For this review, take the finished solid that the model builds, in its own axes (mm). A direction names the side the tool comes from. Round coordinates to 2 decimals unless told otherwise and drop trailing zeros. Loops run counter-clockwise (first coordinate to the right, second up) from the corner with the lowest first, then second, coordinate; pieces in that order, holes last.
1) Take a section at D-D (x = 68.5). State the section outline as (y, z) points.
2) Take a section at B-B (z = 8.25). State the section outline as (x, y) points.
3) Tool access review of faces 1 (the flat face through (20.434, 20.28, 4.93)), 2 (the flat face through (64, 100, 5)), 3 (the flat face through (59, 80, 5)): name each direction out of +Z, -Z, +X, -X, +Y, -Y from which nothing blocks a thin tool from reaching the whole face with its end or side.
4) Take a section at C-C (y = 34). State the section outline as (x, z) points.
5) Mouldability with a two-part tool opening along Y and no side actions: class faces 4 (the flat face through (49, 51, 10)), 5 (the flat face through (8, 0, 5)), 6 (the flat face through (33.72, 69.86, 4.93)) as pulls with the +Y half, pulls with the -Y half, needs draft (parallel to the pull), parting line crosses it, or undercut.
6) Take a section at A-A (x = 55.5). State the section outline as (y, z) points, then the cut area to 3 significant figures.
7) Insertion check: pin 1 (6 mm diameter, centred on x = 59.5, z = 1, fed in from -Y); pin 2 (1.5 mm diameter, centred on y = 64.5, z = 4.5, fed in from +X); pin 3 (1 mm diameter, centred on y = 57, z = 5.5, fed in from -X). Each pin has a flat end and moves straight along its axis. Give the tip position at first contact, or say it passes through.
8) Wall thickness on L1, parallel to Y at x = 46, z = 8.5; L2, parallel to Y at x = 73.5, z = 7.75; L3, parallel to X at y = 75, z = 3.5: over which ranges is each line inside the solid? List them lowest first.
```python
from build123d import *

# Parameters (mm, degrees)
EXTRUDE_A_DEPTH = 10


with BuildPart() as part:
    # Skica5 → A_ (new body)
    with BuildSketch(Plane.XY):
        Polygon((0, 0), (21.435935394, 80), (41.794919243, 100), (86.794919243, 100), (96.435935394, 80), (75, 0), (60, 0), (70.717967697, 40), (25.717967697, 40), (15, 0), align=None)
        Polygon((36.435935394, 80), (81.435935394, 80), (76.076951546, 60), (31.076951546, 60), align=None, mode=Mode.SUBTRACT)
    extrude(amount=EXTRUDE_A_DEPTH)


solid = part.part
```
Response:
1. outline: (0, 0) - (31.72, 0) - (31.72, 10) - (0, 10) - close; (40, 0) - (60, 0) - (60, 10) - (40, 10) - close; (80, 0) - (100, 0) - (100, 10) - (80, 10) - close
2. outline: (0, 0) - (15, 0) - (25.72, 40) - (70.72, 40) - (60, 0) - (75, 0) - (96.44, 80) - (86.79, 100) - (41.79, 100) - (21.44, 80) - close; hole (31.08, 60) - (76.08, 60) - (81.44, 80) - (36.44, 80) - close
3. face 1: +Z, -Z, -Y
3. face 2: +Z, -Z, +X, -X, +Y
3. face 3: +Z, -Z
4. outline: (9.11, 0) - (24.11, 0) - (24.11, 10) - (9.11, 10) - close; (69.11, 0) - (84.11, 0) - (84.11, 10) - (69.11, 10) - close
5. face 4: needs draft
5. face 5: pulls with the -Y half
5. face 6: undercut
6. outline: (40, 0) - (60, 0) - (60, 10) - (40, 10) - close; (80, 0) - (100, 0) - (100, 10) - (80, 10) - close
6. area: 400 mm2
7. pin 1: stops at y = 0
7. pin 2: stops at x = 92.48
7. pin 3: stops at x = 15.14
8. L1: y = 40 to 60, 80 to 100
8. L2: y = 0 to 60, 80 to 100
8. L3: x = 20.1 to 35.1, 80.1 to 95.1
